Design review of the part shown in the three views and the two pictorial views. Dimensions are in mm from the part's minimum x, y and z. Coordinates: 2 decimals unless noted, no trailing zeros. Order: outer loops, then holes, each group sorted by start corner. A loop starts at its lowest first (then second) coordinate and runs counter-clockwise, first axis right, second up. Notation, with made-up numbers: M 2,23 L 26,23 A16 cw 26,37 Z; hole C 11.25,81.25 d1. An arc over 180 degrees is marked long. Use CSV: the item, a comma, the result in double quotes.
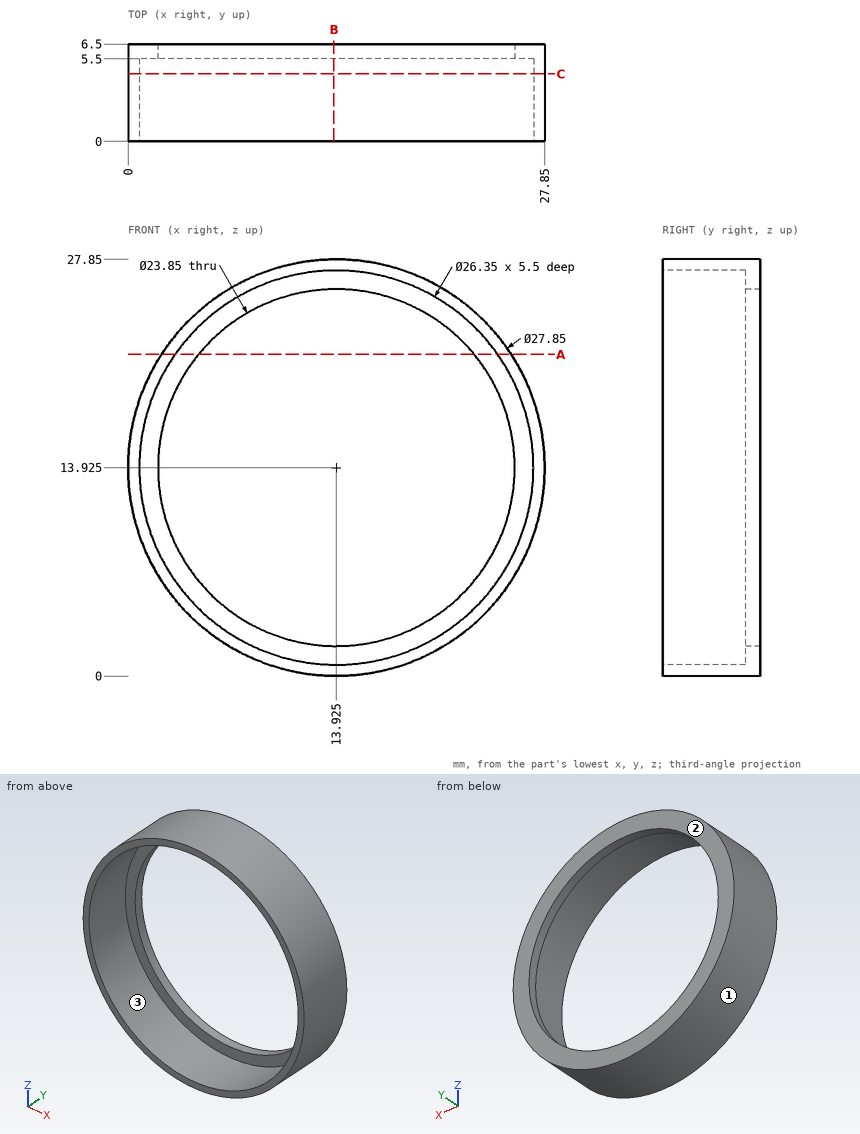
(1) Add section A-A on z = 21.5. State the section outline as (x, y) points.
The answers:
outline,"M 2.24,0 L 3.15,0 L 3.15,5.5 L 4.71,5.5 L 4.71,6.5 L 2.24,6.5 Z; M 23.14,5.5 L 24.7,5.5 L 24.7,0 L 25.61,0 L 25.61,6.5 L 23.14,6.5 Z"
(2) Add section C-C on y = 4.5. State the section outline as (x, z) points (3 decimals).
The answers:
outline,"C 13.925,13.925 d27.85; hole C 13.925,13.925 d26.35"
(3) Clearance check with flat-ended pins moving along their axes: P1, Ø8, axis at x = 16.5, z = 18.5, coming from the -Y side; P2, Ø3, axis at x = 4, y = 2, coming from the +Z side; P3, Ø3, axis at y = 0.5, z = 17.5, coming from the -X side. State where each tip first meets the part, or that it passes through.
The answers:
P1,"passes through"
P2,"stops at z = 25.01"
P3,"stops at x = 0.16"
(4) Wall thickness on probe 1 along X at (y, z) = (3, 11); probe 2 along Z at (x, y) = (6.25, 2); probe 3 along Z at (x, y) = (5, 3.5): over which ranges is each line inside the solid? List them lowest first.
The answers:
probe 1,"x = 0.31 to 1.08, 26.77 to 27.54"
probe 2,"z = 2.31 to 3.22, 24.63 to 25.54"
probe 3,"z = 3.24 to 4.23, 23.62 to 24.61"
(5) The part is to be moulded in two halves that separate along Z. For the marked faces 1, 2 and 3, say which applies: pulls with the +Z half, pulls with the -Z half, needs draft (parallel to the pull), parting line crosses it, or undercut.
The answers:
face 1,"parting line crosses it"
face 2,"needs draft"
face 3,"undercut"
(6) Add section B-B on x = 13.75. State the section outline as (y, z) points, and give its area (3 significant figures).
The answers:
outline,"M 0,0 L 6.5,0 L 6.5,2 L 5.5,2 L 5.5,0.75 L 0,0.75 Z; M 0,27.1 L 5.5,27.1 L 5.5,25.85 L 6.5,25.85 L 6.5,27.85 L 0,27.85 Z"
area,"12.3 mm2"
